from build123d import *

# Parameters (mm, degrees)
SKETCH2_W                    = 223.798385104
SKETCH2_H                    = 130.999439424
TOP_PLATE_DEPTH              = 6.35
PRIMARY_BUTTON_CUTOUTS_REACH = 159.391
BUTTON_CUTOUTS_R             = 12.5
BUTTON_CUTOUTS_R_2           = 15.5
FILLET1_R                    = 1.5
EXTRA_BUTTONS_REACH          = 159.391
SKETCH3_R                    = 2
SKETCH4_W                    = 207.798385104
SKETCH4_H                    = 114.999439424
CUT_EXTRUDE2_DEPTH           = 3.3
SKETCH5_W                    = 14
SKETCH5_H                    = 8
CUT_EXTRUDE3_DEPTH           = 3.3
M3X0_5_TAPPED_HOLE1_D        = 2.5
M3X0_5_TAPPED_HOLE1_DEPTH    = 2.5
M3X0_5_TAPPED_HOLE1_TIP      = 0.751075774
FILLET2_R                    = 1.5


with BuildPart() as part:
    # Sketch2 → top plate (new body)
    with BuildSketch(Plane(origin=(0, 0, 0), x_dir=(1, 0, 0), z_dir=(0, 1, 0))):
        with Locations((0, 44.999719712)):
            Rectangle(SKETCH2_W, SKETCH2_H)
    extrude(amount=TOP_PLATE_DEPTH)

    # Button Cutouts → primary button cutouts (cut, up to next)
    with BuildSketch(Plane(origin=(0, 0, 0), x_dir=(1, 0, 0), z_dir=(0, 1, 0)), mode=Mode.PRIVATE) as primary_button_cutouts_sk1:
        with Locations(Location((24.5, 32, 0), (0, 0, 270))):
            Circle(BUTTON_CUTOUTS_R)
    primary_button_cutouts_tool1 = extrude(primary_button_cutouts_sk1.sketch, amount=PRIMARY_BUTTON_CUTOUTS_REACH, mode=Mode.PRIVATE) & part.part
    # Button Cutouts → primary button cutouts (cut, up to next)
    with BuildSketch(Plane(origin=(0, 0, 0), x_dir=(1, 0, 0), z_dir=(0, 1, 0)), mode=Mode.PRIVATE) as primary_button_cutouts_sk2:
        with Locations(Location((24.5, 61, 0), (0, 0, 270))):
            Circle(BUTTON_CUTOUTS_R)
    primary_button_cutouts_tool2 = extrude(primary_button_cutouts_sk2.sketch, amount=PRIMARY_BUTTON_CUTOUTS_REACH, mode=Mode.PRIVATE) & part.part
    # Button Cutouts → primary button cutouts (cut, up to next)
    with BuildSketch(Plane(origin=(0, 0, 0), x_dir=(1, 0, 0), z_dir=(0, 1, 0)), mode=Mode.PRIVATE) as primary_button_cutouts_sk3:
        with Locations(Location((49.5, 46, 0), (0, 0, 270))):
            Circle(BUTTON_CUTOUTS_R)
    primary_button_cutouts_tool3 = extrude(primary_button_cutouts_sk3.sketch, amount=PRIMARY_BUTTON_CUTOUTS_REACH, mode=Mode.PRIVATE) & part.part
    # Button Cutouts → primary button cutouts (cut, up to next)
    with BuildSketch(Plane(origin=(0, 0, 0), x_dir=(1, 0, 0), z_dir=(0, 1, 0)), mode=Mode.PRIVATE) as primary_button_cutouts_sk4:
        with Locations(Location((49.5, 75, 0), (0, 0, 270))):
            Circle(BUTTON_CUTOUTS_R)
    primary_button_cutouts_tool4 = extrude(primary_button_cutouts_sk4.sketch, amount=PRIMARY_BUTTON_CUTOUTS_REACH, mode=Mode.PRIVATE) & part.part
    # Button Cutouts → primary button cutouts (cut, up to next)
    with BuildSketch(Plane(origin=(0, 0, 0), x_dir=(1, 0, 0), z_dir=(0, 1, 0)), mode=Mode.PRIVATE) as primary_button_cutouts_sk5:
        with Locations(Location((78.5, 75, 0), (0, 0, 270))):
            Circle(BUTTON_CUTOUTS_R)
    primary_button_cutouts_tool5 = extrude(primary_button_cutouts_sk5.sketch, amount=PRIMARY_BUTTON_CUTOUTS_REACH, mode=Mode.PRIVATE) & part.part
    # Button Cutouts → primary button cutouts (cut, up to next)
    with BuildSketch(Plane(origin=(0, 0, 0), x_dir=(1, 0, 0), z_dir=(0, 1, 0)), mode=Mode.PRIVATE) as primary_button_cutouts_sk6:
        with Locations(Location((78.5, 46, 0), (0, 0, 270))):
            Circle(BUTTON_CUTOUTS_R)
    primary_button_cutouts_tool6 = extrude(primary_button_cutouts_sk6.sketch, amount=PRIMARY_BUTTON_CUTOUTS_REACH, mode=Mode.PRIVATE) & part.part
    # Button Cutouts → primary button cutouts (cut, up to next)
    with BuildSketch(Plane(origin=(0, 0, 0), x_dir=(1, 0, 0), z_dir=(0, 1, 0)), mode=Mode.PRIVATE) as primary_button_cutouts_sk7:
        with Locations(Location((-89.899192552, 66.691534373, 0), (0, 0, 270))):
            Circle(BUTTON_CUTOUTS_R_2)
    primary_button_cutouts_tool7 = extrude(primary_button_cutouts_sk7.sketch, amount=PRIMARY_BUTTON_CUTOUTS_REACH, mode=Mode.PRIVATE) & part.part
    # Button Cutouts → primary button cutouts (cut, up to next)
    with BuildSketch(Plane(origin=(0, 0, 0), x_dir=(1, 0, 0), z_dir=(0, 1, 0)), mode=Mode.PRIVATE) as primary_button_cutouts_sk8:
        with Locations(Location((24.680313923, 89.999439424, 0), (0, 0, 270))):
            Circle(BUTTON_CUTOUTS_R)
    primary_button_cutouts_tool8 = extrude(primary_button_cutouts_sk8.sketch, amount=PRIMARY_BUTTON_CUTOUTS_REACH, mode=Mode.PRIVATE) & part.part
    # Button Cutouts → primary button cutouts (cut, up to next)
    with BuildSketch(Plane(origin=(0, 0, 0), x_dir=(1, 0, 0), z_dir=(0, 1, 0)), mode=Mode.PRIVATE) as primary_button_cutouts_sk9:
        with Locations(Location((-0.524094275, 75.65587615, 0), (0, 0, 270))):
            Circle(BUTTON_CUTOUTS_R)
    primary_button_cutouts_tool9 = extrude(primary_button_cutouts_sk9.sketch, amount=PRIMARY_BUTTON_CUTOUTS_REACH, mode=Mode.PRIVATE) & part.part
    # Button Cutouts → primary button cutouts (cut, up to next)
    with BuildSketch(Plane(origin=(0, 0, 0), x_dir=(1, 0, 0), z_dir=(0, 1, 0)), mode=Mode.PRIVATE) as primary_button_cutouts_sk10:
        with BuildLine():
            Line((17.5, -12.5), (-17.5, -12.5))
            ThreePointArc((-17.5, -12.5), (-30, 0), (-17.5, 12.5))
            Line((-17.5, 12.5), (17.5, 12.5))
            ThreePointArc((17.5, 12.5), (30, 0), (17.5, -12.5))
        make_face()
    primary_button_cutouts_tool10 = extrude(primary_button_cutouts_sk10.sketch, amount=PRIMARY_BUTTON_CUTOUTS_REACH, mode=Mode.PRIVATE) & part.part
    # Button Cutouts → primary button cutouts (cut, up to next)
    with BuildSketch(Plane(origin=(0, 0, 0), x_dir=(1, 0, 0), z_dir=(0, 1, 0)), mode=Mode.PRIVATE) as primary_button_cutouts_sk11:
        Polygon((-70.006364371, 68.006025513), (-62.024315273, 85.24803503), (-44.736932046, 77.244980539), (-36.733877555, 94.532363766), (-19.491868038, 86.550314667), (-29.175353919, 65.6330347), (-11.887970692, 57.629980209), (-19.870019791, 40.387970692), (-37.112029308, 48.370019791), (-35.431597919, 51.999916531), align=None)
    primary_button_cutouts_tool11 = extrude(primary_button_cutouts_sk11.sketch, amount=PRIMARY_BUTTON_CUTOUTS_REACH, mode=Mode.PRIVATE) & part.part
    add(primary_button_cutouts_tool1.solids().sort_by_distance((24.5, 0, -32))[0], mode=Mode.SUBTRACT)
    add(primary_button_cutouts_tool2.solids().sort_by_distance((24.5, 0, -61))[0], mode=Mode.SUBTRACT)
    add(primary_button_cutouts_tool3.solids().sort_by_distance((49.5, 0, -46))[0], mode=Mode.SUBTRACT)
    add(primary_button_cutouts_tool4.solids().sort_by_distance((49.5, 0, -75))[0], mode=Mode.SUBTRACT)
    add(primary_button_cutouts_tool5.solids().sort_by_distance((78.5, 0, -75))[0], mode=Mode.SUBTRACT)
    add(primary_button_cutouts_tool6.solids().sort_by_distance((78.5, 0, -46))[0], mode=Mode.SUBTRACT)
    add(primary_button_cutouts_tool7.solids().sort_by_distance((-89.899193, 0, -66.691534))[0], mode=Mode.SUBTRACT)
    add(primary_button_cutouts_tool8.solids().sort_by_distance((24.680314, 0, -89.999439))[0], mode=Mode.SUBTRACT)
    add(primary_button_cutouts_tool9.solids().sort_by_distance((-0.524094, 0, -75.655876))[0], mode=Mode.SUBTRACT)
    add(primary_button_cutouts_tool10.solids().sort_by_distance((0, 0, 0))[0], mode=Mode.SUBTRACT)
    add(primary_button_cutouts_tool11.solids().sort_by_distance((-38.528194, 0, -68.046357))[0], mode=Mode.SUBTRACT)

    # Fillet1
    fillet1_edges = [part.edges().sort_by_distance(p)[0] for p in [
        (-19.491868038, 3.175, -86.550314667),
        (-36.733877555, 3.175, -94.532363766),
        (-62.024315273, 3.175, -85.24803503),
        (-70.006364371, 3.175, -68.006025513),
        (-37.112029308, 3.175, -48.370019791),
        (-19.870019791, 3.175, -40.387970692),
        (-11.887970692, 3.175, -57.629980209),
    ]]
    fillet(fillet1_edges, radius=FILLET1_R)

    # Sketch3 → extra buttons (cut, up to next)
    with BuildSketch(Plane(origin=(0, 6.35, 0), x_dir=(1, 0, 0), z_dir=(0, 1, 0)), mode=Mode.PRIVATE) as extra_buttons_sk1:
        with Locations(Location((50.473746808, 97.976443239, 0), (0, 0, 270))):
            Circle(SKETCH3_R)
    extra_buttons_tool1 = extrude(extra_buttons_sk1.sketch, amount=-EXTRA_BUTTONS_REACH, mode=Mode.PRIVATE) & part.part
    # Sketch3 → extra buttons (cut, up to next)
    with BuildSketch(Plane(origin=(0, 6.35, 0), x_dir=(1, 0, 0), z_dir=(0, 1, 0)), mode=Mode.PRIVATE) as extra_buttons_sk2:
        with Locations(Location((60.473746808, 97.976443239, 0), (0, 0, 270))):
            Circle(SKETCH3_R)
    extra_buttons_tool2 = extrude(extra_buttons_sk2.sketch, amount=-EXTRA_BUTTONS_REACH, mode=Mode.PRIVATE) & part.part
    # Sketch3 → extra buttons (cut, up to next)
    with BuildSketch(Plane(origin=(0, 6.35, 0), x_dir=(1, 0, 0), z_dir=(0, 1, 0)), mode=Mode.PRIVATE) as extra_buttons_sk3:
        with Locations(Location((70.473746808, 97.976443239, 0), (0, 0, 270))):
            Circle(SKETCH3_R)
    extra_buttons_tool3 = extrude(extra_buttons_sk3.sketch, amount=-EXTRA_BUTTONS_REACH, mode=Mode.PRIVATE) & part.part
    # Sketch3 → extra buttons (cut, up to next)
    with BuildSketch(Plane(origin=(0, 6.35, 0), x_dir=(1, 0, 0), z_dir=(0, 1, 0)), mode=Mode.PRIVATE) as extra_buttons_sk4:
        with Locations(Location((80.473746808, 97.976443239, 0), (0, 0, 270))):
            Circle(SKETCH3_R)
    extra_buttons_tool4 = extrude(extra_buttons_sk4.sketch, amount=-EXTRA_BUTTONS_REACH, mode=Mode.PRIVATE) & part.part
    # Sketch3 → extra buttons (cut, up to next)
    with BuildSketch(Plane(origin=(0, 6.35, 0), x_dir=(1, 0, 0), z_dir=(0, 1, 0)), mode=Mode.PRIVATE) as extra_buttons_sk5:
        with Locations(Location((90.473746808, 97.976443239, 0), (0, 0, 270))):
            Circle(SKETCH3_R)
    extra_buttons_tool5 = extrude(extra_buttons_sk5.sketch, amount=-EXTRA_BUTTONS_REACH, mode=Mode.PRIVATE) & part.part
    add(extra_buttons_tool1.solids().sort_by_distance((50.473747, 6.35, -97.976443))[0], mode=Mode.SUBTRACT)
    add(extra_buttons_tool2.solids().sort_by_distance((60.473747, 6.35, -97.976443))[0], mode=Mode.SUBTRACT)
    add(extra_buttons_tool3.solids().sort_by_distance((70.473747, 6.35, -97.976443))[0], mode=Mode.SUBTRACT)
    add(extra_buttons_tool4.solids().sort_by_distance((80.473747, 6.35, -97.976443))[0], mode=Mode.SUBTRACT)
    add(extra_buttons_tool5.solids().sort_by_distance((90.473747, 6.35, -97.976443))[0], mode=Mode.SUBTRACT)

    # Sketch4 → Cut-Extrude2 (cut)
    with BuildSketch(Plane.XZ):
        with Locations((0, -44.999719712)):
            Rectangle(SKETCH4_W, SKETCH4_H)
    extrude(amount=-CUT_EXTRUDE2_DEPTH, mode=Mode.SUBTRACT)

    # Sketch5 → Cut-Extrude3 (cut)
    with BuildSketch(Plane.XZ):
        with Locations((0, -106.499439424)):
            Rectangle(SKETCH5_W, SKETCH5_H)
    extrude(amount=-CUT_EXTRUDE3_DEPTH, mode=Mode.SUBTRACT)

    # M3x0.5 Tapped Hole1
    with Locations(Plane(origin=(-107.899192552, 0, -106.499439424), x_dir=(0, 0, -1), z_dir=(0, -1, 0))):
        with Locations((0, 0), (0, 96.899192552), (0, 118.899192552), (0, 215.798385104), (-122.999439424, 215.798385104), (-122.826484666, 107.899192552), (-122.999439424, 0)):
            Hole(M3X0_5_TAPPED_HOLE1_D / 2, depth=M3X0_5_TAPPED_HOLE1_DEPTH)
            with Locations((0, 0, -(M3X0_5_TAPPED_HOLE1_DEPTH + M3X0_5_TAPPED_HOLE1_TIP / 2))):  # 118° drill point
                Cone(0, M3X0_5_TAPPED_HOLE1_D / 2, M3X0_5_TAPPED_HOLE1_TIP, mode=Mode.SUBTRACT)

    # Fillet2
    fillet2_edges = [part.edges().sort_by_distance(p)[0] for p in [
        (111.899192552, 6.35, -44.999719712),
        (0, 6.35, -110.499439424),
        (-111.899192552, 6.35, -44.999719712),
        (-111.899192552, 3.175, -110.499439424),
        (111.899192552, 3.175, -110.499439424),
        (111.899192552, 3.175, 20.5),
        (-111.899192552, 3.175, 20.5),
        (0, 6.35, 20.5),
    ]]
    fillet(fillet2_edges, radius=FILLET2_R)


solid = part.part
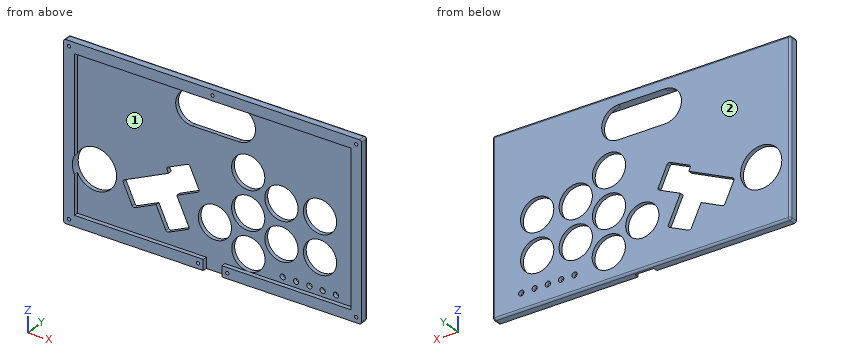
Work out the finished part from the listing and answer in its coordinate system (mm). Face numbers are marked on the shaded views. Round coordinates to 2 decimals unless told otherwise and drop trailing zeros. Loops run counter-clockwise (first coordinate to the right, second up) from the corner with the lowest first, then second, coordinate; pieces in that order, holes last. Notation, with made-up numbers: (29.25, 8.25) - (46.25, 8.25) arc R18 ccw to (46.25, 43.25) - close; hole circle Ø7 at (65.25, 79). An arc over 180 degrees is marked (long way). Use one line per item in the form item = value. Start each with the question number.
(1) Consider line 1 (Z direction, x = 59, y = 2.75); line 2 (X direction, y = 3.25, z = -46); line 3 (X direction, y = 2.5, z = -64.5). Determine where each line is inside the solid, lowest interval first.
(2) Find section A-A on x = 75. Determine the outline of the cut face in (y, z), and give its area (3 significant figures).
(3) Determine the mould class of the marked faces 1 and 2 for opening direction Z: +Z half, -Z half, draft (parallel to the pull), parting line (faces both ways), or undercut.
(4) Find section C-C on z = -9. Determine the outline of the cut face in (x, y).
(5) Find section D-D on x = -82.5. Determine the outline of the cut face in (y, z), and give its area (3 significant figures).
(6) Flat-ended cylindrical pins translate along their axes: P1, Ø10, axis at x = -76.5, z = -63.5, coming from the -Y side; P2, Ø1.5, axis at x = 0, z = 16.33, coming from the -Y side. Find the tip coordinate at first contact, or state that the pin passes through.
(7) Find section B-B on y = 1.5. Determine the outline of the cut face in (x, z), and give its area (3 significant figures).
Answer list:
q1.line_1 = -110.5 to -102.5, 12.5 to 20.5
q1.line_2 = -111.9 to -103.9, 103.9 to 111.9
q1.line_3 = -111.9 to -105.24, 103.9 to 111.9
q2.outline = (0, -110.5) - (4.85, -110.5) arc R1.5 ccw to (6.35, -109) - (6.35, -87) - (3.3, -87) - (3.3, -102.5) - (0, -102.5) - close; (0, 12.5) - (3.3, 12.5) - (3.3, -34) - (6.35, -34) - (6.35, 19) arc R1.5 ccw to (4.85, 20.5) - (0, 20.5) - close; (3.3, -63) - (6.35, -63) - (6.35, -58) - (3.3, -58) - close
q2.area = 305 mm^2
q3.face_1 = undercut
q3.face_2 = draft
q4.outline = (-111.9, 0) - (-103.9, 0) - (-103.9, 3.3) - (-26.17, 3.3) - (-26.17, 6.35) - (-110.4, 6.35) arc R1.5 ccw to (-111.9, 4.85) - close; (26.17, 3.3) - (103.9, 3.3) - (103.9, 0) - (111.9, 0) - (111.9, 4.85) arc R1.5 ccw to (110.4, 6.35) - (26.17, 6.35) - close
q5.outline = (0, -110.5) - (4.85, -110.5) arc R1.5 ccw to (6.35, -109) - (6.35, -80.31) - (3.3, -80.31) - (3.3, -102.5) - (0, -102.5) - close; (0, 12.5) - (3.3, 12.5) - (3.3, -53.07) - (6.35, -53.07) - (6.35, 19) arc R1.5 ccw to (4.85, 20.5) - (0, 20.5) - close
q5.area = 368 mm^2
q6.P1 = 3.3
q6.P2 = 2.8
q7.outline = (-111.9, -109) arc R1.5 ccw to (-110.4, -110.5) - (-7, -110.5) - (-7, -102.5) - (-103.9, -102.5) - (-103.9, -73.34) arc R15.5 cw to (-103.9, -60.04) - (-103.9, 12.5) - (103.9, 12.5) - (103.9, -102.5) - (7, -102.5) - (7, -110.5) - (110.4, -110.5) arc R1.5 ccw to (111.9, -109) - (111.9, 19) arc R1.5 ccw to (110.4, 20.5) - (-110.4, 20.5) arc R1.5 ccw to (-111.9, 19) - close; hole circle Ø2.5 at (-107.9, -106.5); hole circle Ø2.5 at (-107.9, 16.5); hole circle Ø2.5 at (-11, -106.5); hole circle Ø2.5 at (0, 16.33); hole circle Ø2.5 at (11, -106.5); hole circle Ø2.5 at (107.9, -106.5); hole circle Ø2.5 at (107.9, 16.5)
q7.area = 5,260 mm^2
